from build123d import *

# Parameters (mm, degrees)
BOSS_EXTRUDE1_DEPTH   = 10
SKETCH6_R             = 1.75
CUT_EXTRUDE1_DEPTH    = 6
F_2_5MM_DOWEL_HOLE1_D = 2.5
SKETCH9_R             = 1.75
CUT_EXTRUDE2_DEPTH    = 15
F_2_5MM_DOWEL_HOLE2_D = 2.5


with BuildPart() as part:
    # Sketch1 → Boss-Extrude1 (new body)
    with BuildSketch(Plane.XY):
        Polygon((0, 0), (-15, 0), (-15, 18), (-7.5, 18), (-7.5, 8), (0, 8), align=None)
    extrude(amount=BOSS_EXTRUDE1_DEPTH)

    # Sketch6 → Cut-Extrude1 (cut)
    with BuildSketch(Plane(origin=(0, 8, 0), x_dir=(1, 0, 0), z_dir=(0, 1, 0))):
        with Locations(Location((-3.6, -5, 0), (0, 0, 270))):
            Circle(SKETCH6_R)
    extrude(amount=-CUT_EXTRUDE1_DEPTH, mode=Mode.SUBTRACT)

    # Ø2.5mm Dowel Hole1 (through all)
    with Locations(Plane(origin=(0, 2, 0), x_dir=(1, 0, 0), z_dir=(0, 1, 0))):
        with Locations((-3.6, -5)):
            Hole(F_2_5MM_DOWEL_HOLE1_D / 2)

    # Sketch9 → Cut-Extrude2 (cut)
    with BuildSketch(Plane.XZ):
        with Locations(Location((-11.25, 5, 0), (0, 0, 270))):
            Circle(SKETCH9_R)
    extrude(amount=-CUT_EXTRUDE2_DEPTH, mode=Mode.SUBTRACT)

    # Ø2.5mm Dowel Hole2 (through all)
    with Locations(Plane(origin=(0, 15, 0), x_dir=(-1, 0, 0), z_dir=(0, -1, 0))):
        with Locations((11.25, -5)):
            Hole(F_2_5MM_DOWEL_HOLE2_D / 2)


solid = part.part
Can you work these out from the model? Positions are in its coordinate system, mm. A direction names the side the tool comes from. Coordinates: 2 decimals unless noted, no trailing zeros. Loops run counter-clockwise (first coordinate to the right, second up) from the corner with the lowest first, then second, coordinate; pieces in that order, holes last. Notation, with made-up numbers: (80, 87.25) - (91, 87.25) arc R18 ccw to (91, 105.25) - close; hole circle Ø8 at (23, 26). An arc over 180 degrees is marked (long way). Put each result on its own line as item: value. Start each with the question number.
Item 1: Which directions (+Z, -Z, +X, -X, +Y, -Y) give clear straight access to the entire face, cutting with the end or side of a thin tool? Please do faces 1 (the face through (0, 4, 5)), 2 (the face through (-7.5, 13, 5)), 3 (the face through (-9.515, 7.395, 5.228)), 4 (the face through (-3.52, 5.04, 3.25)).
Item 2: If I drill on line 1 along X through (y, z) = (3.35, 5); line 2 along X through (y, z) = (1.4, 5); line 3 along Z through (x, y) = (-11.25, 16.75), over which ranges is the centre line in solid material (lowest first)?
Item 3: For pin 1 (2 mm diameter, centred on x = -4, z = 5, fed in from +Y); pin 2 (4 mm diameter, centred on x = -3, z = 5, fed in from +Y); pin 3 (3 mm diameter, centred on x = -11.25, z = 5, fed in from -Y), each with a flat end and sliding along its axis, tell me the tip position at first contact or that it passes through.
Item 4: Suppose I cut it at C-C (y = 10.5). Please give me the cut outline in (x, z), and give its area (3 significant figures).
Item 5: If we mould it in two halves opening along X, with no side actions, what happens to faces 5 (the face through (-12.4, 15, 4.2)), 6 (the face through (-4.177, 0.986, 6.109)), 7 (the face through (-15, 9, 5)), 8 (the face through (-5.5, 8, 4.9))? For each: +X half, -X half, draft (parallel to the pull), parting line (faces both ways), or undercut.
Item 6: Suppose I cut it at B-B (x = -11.25). Please give me the cut outline in (y, z), and give its area (3 significant figures).
Item 7: Suppose I cut it at A-A (z = 5). Please give me the cut outline in (x, y), and give its area (3 significant figures).
Item 8: Suppose I cut it at D-D (y = 7.5). Please give me the cut outline in (x, z).
Here are the results:
1. face 1: +Z, -Z, +X, +Y, -Y
1. face 2: +Z, -Z, +X, +Y
1. face 3: -Y
1. face 4: +Y
2. line 1: -15 to -13, -9.5 to -5.35, -1.85 to 0
2. line 2: -15 to -13, -9.5 to -4.85, -2.35 to 0
2. line 3: 0 to 3.75, 6.25 to 10
3. pin 1: y = 2
3. pin 2: y = 8
3. pin 3: y = 15
4. outline: (-15, 0) - (-7.5, 0) - (-7.5, 10) - (-15, 10) - close; hole circle Ø3.5 at (-11.25, 5)
4. area: 65.4 mm²
5. face 5: undercut
5. face 6: undercut
5. face 7: -X half
5. face 8: draft
6. outline: (0, 0) - (18, 0) - (18, 3.75) - (15, 3.75) - (15, 3.25) - (0, 3.25) - close; (0, 6.75) - (15, 6.75) - (15, 6.25) - (18, 6.25) - (18, 10) - (0, 10) - close
6. area: 120 mm²
7. outline: (-15, 0) - (-13, 0) - (-13, 15) - (-12.5, 15) - (-12.5, 18) - (-15, 18) - close; (-10, 15) - (-9.5, 15) - (-9.5, 0) - (-4.85, 0) - (-4.85, 2) - (-5.35, 2) - (-5.35, 8) - (-7.5, 8) - (-7.5, 18) - (-10, 18) - close; (-2.35, 0) - (0, 0) - (0, 8) - (-1.85, 8) - (-1.85, 2) - (-2.35, 2) - close
7. area: 109 mm²
8. outline: (-15, 0) - (0, 0) - (0, 10) - (-15, 10) - close; hole circle Ø3.5 at (-11.25, 5); hole circle Ø3.5 at (-3.6, 5)
